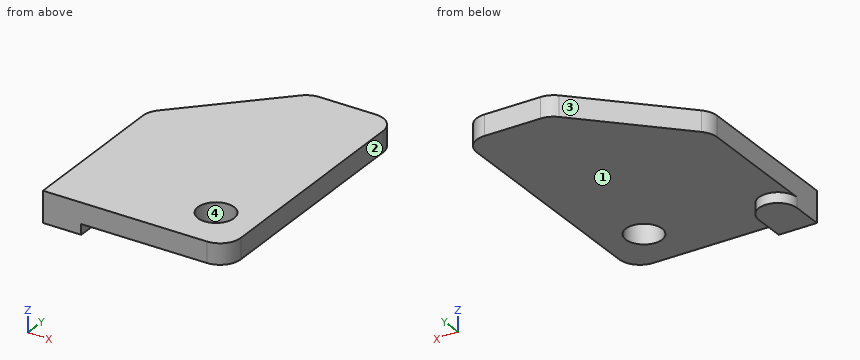
Autodesk Inventor part; units mm, degrees
ref_plane "YZ Plane" through (0, 0, 0) normal (1, 0, 0) x (0, 1, 0)
ref_plane "XZ Plane" through (0, 0, 0) normal (0, 1, 0) x (-1, 0, 0)
ref_plane "XY Plane" through (0, 0, 0) normal (0, 0, 1) x (1, 0, 0)
sketch "Sketch1" plane through (0, 0, 0) normal (0, 0, 1) x (1, 0, 0)
  line L0 (0, 0) -> (0, 25.452)
  line L1 (0, 25.452) -> (-8.276, 25.452)
  line L2 (-8.276, 25.452) -> (-18, 15.728)
  line L3 (-18, 15.728) -> (-18, 0)
  line L4 (-18, 0) -> (0, 0)
  dimension "d0" = 8.276
  dimension "d1" = 18
  dimension "d2" = 135
  dimension "d3" = 25.452
extrude "Extrusion1" add sketch "Sketch1" along normal blind 2
sketch "Sketch2" plane through (0, 0, 2) normal (0, 0, 1) x (1, 0, 0)
  line L0 (0, 25.452) -> (-8.276, 25.452)
  line L1 (-8.276, 25.452) -> (-18, 15.728)
  line L2 (-18, 15.728) -> (-18, 0)
  line L3 (-18, 0) -> (0, 0)
  line L4 (0, 0) -> (0, 25.452)
  line L5 (-18, 0) -> (0, 0)
  line L6 (-14, 0) -> (-14, 3)
  arc A0 (-14, 3) -> (-18, 3) centre (-16, 3) ccw
  dimension "d6" = 4
  dimension "d7" = 3
  dimension "d8" = 2
extrude "Extrusion2" add sketch "Sketch2" against normal blind 3 contours L3 L2 A0 L6
sketch "Sketch7" plane through (0, 0, -1) normal (0, 0, -1) x (-1, 0, 0)
  line L0 (18, 0) -> (18, 3)
  arc A0 (18, 3) -> (14, 3) centre (16, 3) ccw
  line L1 (14, 3) -> (14, 0)
  line L2 (14, 0) -> (18, 0)
  arc A1 (17.85, 3) -> (14.15, 3) centre (16, 3) ccw
  line L3 (17.85, 3) -> (17.85, 0.15)
  line L4 (17.85, 0.15) -> (14.15, 0.15)
  line L5 (14.15, 0.15) -> (14.15, 3)
  line L6 (14.15, 0.15) -> (14.15, 0)
  line L7 (17.85, 0.15) -> (17.85, 0)
  point P0 (0, 0)
  dimension "d24" = 0.15
extrude "Extrusion6" cut sketch "Sketch7" against normal up to surface (1 mm away) contours L2 L7 L3 A1 L5 L6 L1 A0 L0
sketch "Sketch4" plane through (0, 0, 2) normal (0, 0, 1) x (1, 0, 0)
  circle A0 centre (-4, 4.5) radius 1.75
  line L0 (-18, 15.728) -> (-18, 0)
  line L1 (-18, 0) -> (0, 0)
  point P0 (-14.15, 0)
  point P1 (-18, 3)
  point P2 (-14, 0)
  dimension "d14" = 3.5
  dimension "d15" = 14
  dimension "d16" = 4.5
extrude "Extrusion4" cut sketch "Sketch4" against normal up to surface (2 mm away)
sketch "Sketch5" plane through (-18, 0, 0) normal (-1, 0, 0) x (0, 0, 1)
  line L0 (2, 15.728) -> (2, 0)
  line L1 (0, 15.728) -> (2, 15.728)
  line L2 (2, 0) -> (2, 25.452)
  line L3 (0, 15.728) -> (2, 15.728)
  line L4 (2, 15.728) -> (2, 19.0295)
  line L5 (2, 19.0295) -> (0, 19.0295)
  line L6 (0, 19.0295) -> (0, 15.728)
  line L7 (0, 15.728) -> (0, 0)
  line L8 (0, 0) -> (2, 0)
  point P0 (0, 0)
extrude "Extrusion5" cut sketch "Sketch5" against normal up to surface (0.15 mm away)
fillet "Fillet1" radius 2 4 edges at (-8.276, 25.452, 1) (-17.85, 15.878, 1) (0, 25.452, 1) (0, 0, 1)
sketch "Sketch6" plane through (0, 0, 2) normal (0, 0, 1) x (1, 0, 0)
  circle A0 centre (1.75, 1.9974) radius 1.5
  line L0 (0, 2) -> (0, 23.452)
  point P0 (0, 0)
  dimension "d22" = 3
  dimension "d23" = 1.75
properties part number "ScrewStopper"
Part model, mm, in its own coordinate system. Face numbers are marked on the shaded views. Give positions to 0.01 mm unless a question says otherwise; leave off trailing zeros. Loops run counter-clockwise (first coordinate to the right, second up) from the corner with the lowest first, then second, coordinate; pieces in that order, holes last.
(1) Band-saw the part on A-A (x = -4). Write the cut outline in (y, z), and give its area (3 significant figures).
Return value:
outline: (0, 0) - (2.75, 0) - (2.75, 2) - (0, 2) - close; (6.25, 0) - (25.45, 0) - (25.45, 2) - (6.25, 2) - close
area: 43.9 mm2
(2) Band-saw the part on D-D (y = 10.75). Write the cut outline in (x, z), and give its area (3 significant figures).
Return value:
outline: (-17.85, 0) - (0, 0) - (0, 2) - (-17.85, 2) - close
area: 35.7 mm2
(3) Pull direction X, two halves, no side cores. Call the marked faces 1, 2, 3 and 4: pulls with the +X half, pulls with the -X half, needs draft (parallel to the pull), parting line crosses it, or undercut.
Return value:
face 1: needs draft
face 2: pulls with the +X half
face 3: pulls with the -X half
face 4: undercut
(4) Drill centre lines: line 1 along Y through (x, z) = (-4, 1.6); line 2 along Z through (x, y) = (-4, 1.5); line 3 along Y through (x, z) = (-10.5, 0.6). Where is each one in solid material? Low to high.
Return value:
line 1: y = 0 to 2.75, 6.25 to 25.45
line 2: z = 0 to 2
line 3: y = 0 to 23.23
(5) Pin check, flat tips, straight feed: pin 1 (1.5 mm diameter, centred on y = 12, z = 1.5, fed in from +X); pin 2 (1.5 mm diameter, centred on x = -13, y = 16.5, fed in from -Z); pin 3 (1.5 mm diameter, centred on x = -11, z = 1.5, fed in from +Y). Stop position of each tip, or through.
Return value:
pin 1: stops at x = 0
pin 2: stops at z = 0
pin 3: stops at y = 23.48
(6) Band-saw the part on B-B (z = 1.3). Write the cut outline in (x, y), and give its area (3 significant figures).
Return value:
outline: (-17.85, 0) - (-2, 0) arc R2 ccw to (0, 2) - (0, 23.45) arc R2 ccw to (-2, 25.45) - (-7.45, 25.45) arc R2 ccw to (-8.86, 24.87) - (-17.26, 16.46) arc R2 ccw to (-17.85, 15.05) - close; hole circle Ø3.5 at (-4, 4.5)
area: 397 mm2
